from build123d import *

# Parameters (mm, degrees)
SCHIZZO1_W                   = 80
SCHIZZO1_H                   = 8
SCHIZZO1_R                   = 2.25
SCHIZZO1_R_2                 = 1.85
ESTRUSIONE_ESTRUSIONE1_DEPTH = 5
SCHIZZO2_W                   = 20
SCHIZZO2_H                   = 4
TAGLIO_ESTRUSIONE1_DEPTH     = 8


with BuildPart() as part:
    # Schizzo1 → Estrusione-Estrusione1 (new body)
    with BuildSketch(Plane.XY):
        Rectangle(SCHIZZO1_W, SCHIZZO1_H)
        with Locations((-36, 0)):
            Circle(SCHIZZO1_R, mode=Mode.SUBTRACT)
        Circle(SCHIZZO1_R_2, mode=Mode.SUBTRACT)
        with Locations((36, 0)):
            Circle(SCHIZZO1_R, mode=Mode.SUBTRACT)
    extrude(amount=ESTRUSIONE_ESTRUSIONE1_DEPTH)

    # Schizzo2 → Taglio-Estrusione1 (cut)
    with BuildSketch(Plane.XY.offset(5)):
        with Locations((20, -2)):
            Rectangle(SCHIZZO2_W, SCHIZZO2_H)
    extrude(amount=-TAGLIO_ESTRUSIONE1_DEPTH, mode=Mode.SUBTRACT)


solid = part.part
Read the model definition and answer for the solid it produces. Units are mm, in the model's axes. A direction names the side the tool comes from. Give positions to 0.01 mm unless a question says otherwise; leave off trailing zeros. Write each loop counter-clockwise with the first axis right and the second up, starting at its lowest first coordinate (ties: lowest second). Pieces come first, ordered by that corner, then holes. Notation, with made-up numbers: (62, -29.5) - (75, -29.5) arc R4 cw to (75, -25.5) - close; hole circle Ø6 at (35, 10). An arc over 180 degrees is marked (long way). Return JSON: item names as keys, results as strings.
Q1. A cutting plane is placed at A-A, the plane z = 4.25. Determine the outline of the cut face in (x, y).
Reply:
{"outline": "(-40, -4) - (10, -4) - (10, 0) - (30, 0) - (30, -4) - (40, -4) - (40, 4) - (-40, 4) - close; hole circle Ø4.5 at (-36, 0); hole circle Ø3.7 at (0, 0); hole circle Ø4.5 at (36, 0)"}
Q2. Consider line 1 along Y through (x, z) = (-36, 2.85); line 2 along X through (y, z) = (0.5, 3.35); line 3 along X through (y, z) = (-0.75, 1.8). Determine where each line is inside the solid, lowest interval first. Write a range as [from, to].
Reply:
{"line 1": "[-4, -2.25], [2.25, 4]", "line 2": "[-40, -38.19], [-33.81, -1.78], [1.78, 33.81], [38.19, 40]", "line 3": "[-40, -38.12], [-33.88, -1.69], [1.69, 10], [30, 33.88], [38.12, 40]"}
Q3. For a pull along X with two mould halves and no side action, classify faces 1 (the face through (-15, -4, 2)), 2 (the face through (30, -2, 3)), 3 (the face through (40, 0, 2)) as released by +X, released by -X, zero draft, split by the parting line, or undercut.
Reply:
{"face 1": "zero draft", "face 2": "undercut", "face 3": "released by +X"}
Q4. A cutting plane is placed at B-B, the plane x = -36. Determine the outline of the cut face in (y, z).
Reply:
{"outline": "(-4, 0) - (-2.25, 0) - (-2.25, 5) - (-4, 5) - close; (2.25, 0) - (4, 0) - (4, 5) - (2.25, 5) - close"}
Q5. Given P1, Ø4, axis at x = 11.5, y = -1.5, coming from the -Z side; P2, Ø2.5, axis at x = 19.5, z = 2.5, coming from the -Y side, each flat-ended and moving along its own axis, determine where each tip first touches the part or whether it passes through.
Reply:
{"P1": "z = 0", "P2": "y = 0"}
Q6. A cutting plane is placed at C-C, the plane x = 0. Determine the outline of the cut face in (y, z).
Reply:
{"outline": "(-4, 0) - (-1.85, 0) - (-1.85, 5) - (-4, 5) - close; (1.85, 0) - (4, 0) - (4, 5) - (1.85, 5) - close"}
Q7. For faces 4 (the face through (-40, 0, 2)), 5 (the face through (10, -2, 3)), determine the directions among +Z, -Z, +X, -X, +Y, -Y from which every point of the face is accessible in a straight line to the end or side of a thin tool.
Reply:
{"face 4": "+Z, -Z, -X, +Y, -Y", "face 5": "+Z, -Z, -Y"}
Q8. A cutting plane is placed at D-D, the plane x = 18. Determine the outline of the cut face in (y, z), and give its area (3 significant figures).
Reply:
{"outline": "(0, 0) - (4, 0) - (4, 5) - (0, 5) - close", "area": "20.0 mm²"}
